Geometry: final body of the model. Coordinates: model frame, mm. A direction names the side the tool comes from. Coordinates: 2 decimals unless noted, no trailing zeros. Write each loop counter-clockwise with the first axis right and the second up, starting at its lowest first coordinate (ties: lowest second). Pieces come first, ordered by that corner, then holes. Notation, with made-up numbers: (2.5, -3) -> (42.5, -3) arc R11 ccw to (42.5, 3) -> close; hole circle Ø4 at (-0.75, 26.5). An arc over 180 degrees is marked (long way). One line per item, written item: value.
```python
from build123d import *

# Parameters (mm, degrees)
CORTE_EXTRUS_O1_DEPTH    = 5
ESBO_O3_W                = 2.513225657
ESBO_O3_H                = 5.478331089
RESSALTO_EXTRUS_O1_DEPTH = 5


with BuildPart() as part:
    # Esboço1 → Revolução1 (revolve)
    with BuildSketch(Plane.XY):
        Polygon((-1, 10), (-5, 10), (-5, 0), (-2, 0), (-2, 5), (-1, 5), align=None)
    revolve(axis=Axis((0, 0, 0), (0, 1, 0)))

    # Esboço2 → Corte-extrusão1 (cut)
    with BuildSketch(Plane(origin=(0, 10, 0), x_dir=(1, 0, 0), z_dir=(0, 1, 0))):
        with BuildLine():
            Line((1.6, 1.788854382), (1.6, -1.788854382))
            ThreePointArc((1.6, -1.788854382), (-2.4, 0), (1.6, 1.788854382))
        make_face()
    extrude(amount=-CORTE_EXTRUS_O1_DEPTH, mode=Mode.SUBTRACT)

    # Esboço3 → Ressalto-extrusão1 (add)
    with BuildSketch(Plane.XZ):
        with Locations((1.756612829, -0.034046623)):
            Rectangle(ESBO_O3_W, ESBO_O3_H)
    extrude(amount=-RESSALTO_EXTRUS_O1_DEPTH)


solid = part.part
```
(1) Section C-C (y = 6.5). Return the cut outline in (x, z).
Responses:
outline: circle Ø10 at (0, 0); hole (1.6, -1.79) -> (1.6, 1.79) arc R2.4 ccw (long way) to start
(2) Pull-direction query (Z, two-part tool) for faces 1 (the cylindrical face through (-2, 3, 0)), 2 (the cylindrical face through (1.08, 4.93, -4.88)), 3 (the flat face through (2, 10, 0)); classes: released by +Z, released by -Z, zero draft, split by the parting line, or undercut.
Responses:
face 1: undercut
face 2: split by the parting line
face 3: zero draft
(3) Section D-D (x = -2.25). Return the cut outline in (y, z), then the cut area to 3 significant figures.
Responses:
outline: (0, -4.47) -> (10, -4.47) -> (10, -0.84) -> (5, -0.84) -> (5, 0.84) -> (10, 0.84) -> (10, 4.47) -> (0, 4.47) -> close
area: 81.0 mm2
(4) First-contact query: pin 1 (1 mm diameter, centred on y = 3, z = -3, fed in from -X); pin 2 (3 mm diameter, centred on y = 3.5, z = -3, fed in from +X); pin 3 (4.5 mm diameter, centred on x = 0, z = 0, fed in from -Y); pin 4 (1.1 mm diameter, centred on y = 8.5, z = 1, fed in from -X). Flat tips, straight axial feed; report the tip coordinate or a pass-through.
Responses:
pin 1: stops at x = -4.33
pin 2: stops at x = 4.77
pin 3: stops at y = 0
pin 4: stops at x = -4.98
(5) Section A-A (x = 0). Return the cut outline in (y, z), then the cut area to 3 significant figures.
Responses:
outline: (0, -5) -> (10, -5) -> (10, -2.4) -> (5, -2.4) -> (5, -2) -> (0, -2) -> close; (0, 2) -> (5, 2) -> (5, 2.4) -> (10, 2.4) -> (10, 5) -> (0, 5) -> close
area: 56.0 mm2
(6) Section B-B (z = 0). Return the cut outline in (x, y), then the cut area to 3 significant figures.
Responses:
outline: (-5, 0) -> (-2, 0) -> (-2, 5) -> (-2.4, 5) -> (-2.4, 10) -> (-5, 10) -> close; (0.5, 0) -> (5, 0) -> (5, 10) -> (1.6, 10) -> (1.6, 5) -> (0.5, 5) -> close
area: 67.5 mm2
(7) Line query: line 1 (Z direction, x = 0, y = 2.1); line 2 (Z direction, x = 0, y = 6.5); line 3 (X direction, y = 2.75, z = -0.75). Output: solid intervals per line, ascending. Write a range as [from, to].
Responses:
line 1: z = [-5, -2], [2, 5]
line 2: z = [-5, -2.4], [2.4, 5]
line 3: x = [-4.94, -1.85], [0.5, 4.94]
(8) Reachability of faces 4 (the flat face through (0.5, 2, 0)), 5 (the flat face through (1.6, 8, 0)), 6 (the flat face through (1, 0, 0)) from +Z, -Z, +X, -X, +Y, -Y: full face, straight path, thin tool, end or side. Return the list, or none.
Responses:
face 4: +Y, -Y
face 5: +Y
face 6: +Z, -Z, +X, -X, -Y
